Could you check a few things on this model? Use its own coordinates, in mm. A direction names the side the tool comes from. Give positions to 0.01 mm unless a question says otherwise; leave off trailing zeros. Loops run counter-clockwise (first coordinate to the right, second up) from the corner with the lowest first, then second, coordinate; pieces in that order, holes last.
1. Imagine slicing it at C-C (y = 28.5). List the corners of the cut face in (x, z) for me (3 decimals).
2. Imagine slicing it at B-B (x = -20.5). List the corners of the cut face in (y, z) for me (3 decimals), plus the area to 3 significant figures.
3. For faces 1 (the flat face through (-28.7, 19.05, -4.4)), 2 (the flat face through (-30.274, 13.525, 5.11)), 3 (the flat face through (-5, -2.381, 1)), which set-ups out of +Z, -Z, +X, -X, +Y, -Y let a thin tool reach every point of the face, with its end or its side?
4. Thinking about a two-plate mould opening in X: for faces 4 (the flat face through (-1, 2, 38.1)), 5 (the flat face through (-19.05, 13, 0)), 6 (the flat face through (-1, 6.35, 1)), 7 (the flat face through (-4.9, -5.46, 0.53)), which applies, +X half, -X half, draft (parallel to the pull), parting line (faces both ways), or undercut?
5. For P1, Ø3, axis at x = 22, z = -8.5, coming from the -Y side; P2, Ø5, axis at x = 34.5, y = 22, coming from the +Z side (3 decimals); P3, Ø6, axis at x = 4, z = -17.5, coming from the -Y side; P4, Ø6.5, axis at x = -27, y = 10.5, coming from the -Z side (3 decimals), each with a flat end and sliding along its axis, tell me the tip position at first contact or that it passes through.
6. I need wall thicknesses on line 1 along X through (y, z) = (13, -1.5) (3 decimals); line 2 along Y through (x, z) = (-14, 10.5). Which ranges of each line are inside material? Lowest first, please.
```python
from build123d import *

# Parameters (mm, degrees)
SKETCH1_W                       = 76.2
SKETCH1_H                       = 6.35
BOSS_EXTRUDE1_DEPTH             = 38.1
SKETCH2_W                       = 19.05
SKETCH2_H                       = 12.7
SKETCH2_W_2                     = 6.35
SKETCH2_H_2                     = 38.1
BOSS_EXTRUDE2_DEPTH             = 9.525
BOSS_EXTRUDE3_REACH             = 71.85
BOSS_EXTRUDE3_DIRECTION_2_REACH = 71.85
CUT_EXTRUDE2_START              = 38.1
CUT_EXTRUDE2_DEPTH              = 15.875
FILLET1_R                       = 0.508


with BuildPart() as part:
    # Sketch1 → Boss-Extrude1 (new, symmetric)
    with BuildSketch(Plane.XY):
        with Locations((0, 3.175)):
            Rectangle(SKETCH1_W, SKETCH1_H)
    extrude(amount=BOSS_EXTRUDE1_DEPTH, both=True)

    # Sketch2 → Boss-Extrude2 (add, symmetric)
    with BuildSketch(Plane.XY):
        with Locations((-28.575, 12.7)):
            Rectangle(SKETCH2_W, SKETCH2_H)
        with Locations((34.925, 25.4)):
            Rectangle(SKETCH2_W_2, SKETCH2_H_2)
    extrude(amount=BOSS_EXTRUDE2_DEPTH, both=True)

    # Boss-Extrude3: up to this face of the body (flat: up to its plane)
    boss_extrude3_end = Plane(part.part.faces().sort_by_distance((0, 3.175, 38.1))[0])
    # Sketch3 → Boss-Extrude3 (add, up to the picked face)
    with BuildSketch(Plane.XY, mode=Mode.PRIVATE) as boss_extrude3_sk1:
        Polygon((-3.175, 0), (-3.175, -2.38125), (-7.540625, -2.38125), (-2.778125, -7.9375), (2.778125, -7.9375), (7.540625, -2.38125), (3.175, -2.38125), (3.175, 0), align=None)
    boss_extrude3_tool1 = split(extrude(boss_extrude3_sk1.sketch, amount=BOSS_EXTRUDE3_REACH, mode=Mode.PRIVATE), bisect_by=boss_extrude3_end, keep=Keep.BOTH, mode=Mode.PRIVATE)
    add(boss_extrude3_tool1.solids().sort_by(Axis((0, -3.992908, 0), (0, 0, 1)))[0])

    # Boss-Extrude3 direction 2: up to this face of the body (flat: up to its plane)
    boss_extrude3_direction_2_end = Plane(part.part.faces().sort_by_distance((0, 3.175, -38.1))[0])
    # Sketch3 → Boss-Extrude3 direction 2 (add, up to the picked face)
    with BuildSketch(Plane.XY, mode=Mode.PRIVATE) as boss_extrude3_direction_2_sk1:
        Polygon((-3.175, 0), (-3.175, -2.38125), (-7.540625, -2.38125), (-2.778125, -7.9375), (2.778125, -7.9375), (7.540625, -2.38125), (3.175, -2.38125), (3.175, 0), align=None)
    boss_extrude3_direction_2_tool1 = split(extrude(boss_extrude3_direction_2_sk1.sketch, amount=-BOSS_EXTRUDE3_DIRECTION_2_REACH, mode=Mode.PRIVATE), bisect_by=boss_extrude3_direction_2_end, keep=Keep.BOTH, mode=Mode.PRIVATE)
    add(boss_extrude3_direction_2_tool1.solids().sort_by(Axis((0, -3.992908, 0), (0, 0, -1)))[0])

    # Sketch5 → Cut-Extrude2 (cut)
    with BuildSketch(Plane.ZY.offset(CUT_EXTRUDE2_START)):
        Polygon((-3.375, 19.05), (-3.375, 16.86875), (-7.975469127, 16.86875), (-2.870111984, 10.9125), (2.870111984, 10.9125), (7.975469127, 16.86875), (3.375, 16.86875), (3.375, 19.05), align=None)
    extrude(amount=-CUT_EXTRUDE2_DEPTH, mode=Mode.SUBTRACT)

    # Fillet1
    fillet1_edges = [part.edges().sort_by_distance(p)[0] for p in [
        (3.175, 0, 0),
        (-3.175, 0, 0),
        (-3.175, -2.38125, 0),
        (-7.540625, -2.38125, 0),
        (-2.778125, -7.9375, 0),
        (2.778125, -7.9375, 0),
        (7.540625, -2.38125, 0),
        (3.175, -2.38125, 0),
        (-30.1625, 19.05, -3.375),
        (-30.1625, 19.05, 3.375),
        (-30.1625, 16.86875, 3.375),
        (-30.1625, 16.86875, 7.975469127),
        (-30.1625, 10.9125, 2.870111984),
        (-30.1625, 10.9125, -2.870111984),
        (-30.1625, 16.86875, -7.975469127),
        (-30.1625, 16.86875, -3.375),
    ]]
    fillet(fillet1_edges, radius=FILLET1_R)


solid = part.part
```
Derived:
1. outline: (31.75, -9.525) - (38.1, -9.525) - (38.1, 9.525) - (31.75, 9.525) - close
2. outline: (0, -38.1) - (6.35, -38.1) - (6.35, -9.525) - (19.05, -9.525) - (19.05, 9.525) - (6.35, 9.525) - (6.35, 38.1) - (0, 38.1) - close
2. area: 726 mm2
3. face 1: +Z, -Z, -X, +Y
3. face 2: -X
3. face 3: +Z, -Z, -X
4. face 4: draft
4. face 5: undercut
4. face 6: undercut
4. face 7: -X half
5. P1: stops at y = 0
5. P2: stops at z = 9.525
5. P3: stops at y = -7.94
5. P4: stops at z = -9.525
6. line 1: x = -22.225 to -19.05, 31.75 to 38.1
6. line 2: y = 0 to 6.35
